Geometry: final body of the model. Coordinates: model frame, mm. A direction names the side the tool comes from. Round coordinates to 2 decimals unless told otherwise and drop trailing zeros. Write each loop counter-clockwise with the first axis right and the second up, starting at its lowest first coordinate (ties: lowest second). Pieces come first, ordered by that corner, then holes. Notation, with made-up numbers: (66, 53.25) - (110, 53.25) arc R8 cw to (110, 62.25) - close; hole circle Ø2 at (89, 0.5). An arc over 180 degrees is marked (long way). Write each question's results on one line, items separated by ' | '.
from build123d import *

# Parameters (mm, degrees)
EXTRUDE_1_DEPTH = 0.8
FILLET_1_R      = 4
FILLET_2_R      = 2


with BuildPart() as part:
    # 草图1 → 凸台-拉伸1 (new body)
    with BuildSketch(Plane(origin=(0, 0, 0), x_dir=(1, 0, 0), z_dir=(0, 1, 0))):
        with BuildLine():
            ThreePointArc((1.559359784, 16.778866316), (1.803429124, 18.895886668), (0, 20.03122292))
            Line((0, 20.03122292), (0, 18.83122292))
            ThreePointArc((0, 18.83122292), (0.8, 18.03122292), (0, 17.23122292))
            Line((0, 17.23122292), (0, 15.142135624))
            ThreePointArc((0, 15.142135624), (1, 14.142135624), (0, 13.142135624))
            Line((0, 13.142135624), (0, 12.142135624))
            Line((0, 12.142135624), (7.708712153, 11))
            ThreePointArc((7.708712153, 11), (7.543556444, 9.535365676), (8.232233047, 8.232233047))
            Line((8.232233047, 8.232233047), (9.292893219, 9.292893219))
            ThreePointArc((9.292893219, 9.292893219), (9.292893219, 10.707106781), (10.707106781, 10.707106781))
            Line((10.707106781, 10.707106781), (11.767766953, 11.767766953))
            ThreePointArc((11.767766953, 11.767766953), (9.864121635, 12.496304683), (8.05080027, 11.565445755))
            Line((8.05080027, 11.565445755), (1.559359784, 16.778866316))
        make_face()
    extrude_1 = extrude(amount=EXTRUDE_1_DEPTH)

    # 镜向1: 凸台-拉伸1 across plane
    add(extrude_1.mirror(Plane(origin=(0, 0.8, 0), x_dir=(-0.707106781, 0, 0.707106781), z_dir=(-0.707106781, 0, -0.707106781))))

    # 镜向2: part across plane


with BuildPart() as part_1:
    add(part.part)
    add(part.part.mirror(Plane(origin=(0, 0.8, 0), x_dir=(0, 0, 1), z_dir=(1, 0, 0))))

    # 镜向3: part across plane


with BuildPart() as part_2:
    add(part_1.part)
    add(part_1.part.mirror(Plane(origin=(0, 0.8, 0), x_dir=(1, 0, 0), z_dir=(0, 0, 1))))

    # 圆角1
    fillet_1_edges = [part_2.edges().sort_by_distance(p)[0] for p in [
        (7.708712153, 0.4, 11),
        (11, 0.4, 7.708712153),
        (12.142135624, 0.4, 0),
        (0, 0.4, 12.142135624),
        (-7.708712153, 0.4, 11),
        (-11, 0.4, 7.708712153),
        (-12.142135624, 0.4, 0),
        (7.708712153, 0.4, -11),
        (11, 0.4, -7.708712153),
        (0, 0.4, -12.142135624),
        (-7.708712153, 0.4, -11),
        (-11, 0.4, -7.708712153),
    ]]
    fillet(fillet_1_edges, radius=FILLET_1_R)

    # 圆角2
    fillet_2_edges = [part_2.edges().sort_by_distance(p)[0] for p in [
        (8.05080027, 0.4, 11.565445755),
        (1.559359784, 0.4, 16.778866316),
        (-1.559359784, 0.4, 16.778866316),
        (16.778866316, 0.4, 1.559359784),
        (11.565445755, 0.4, 8.05080027),
        (-11.565445755, 0.4, 8.05080027),
        (-8.05080027, 0.4, 11.565445755),
        (-16.778866316, 0.4, 1.559359784),
        (1.559359784, 0.4, -16.778866316),
        (8.05080027, 0.4, -11.565445755),
        (16.778866316, 0.4, -1.559359784),
        (11.565445755, 0.4, -8.05080027),
        (-8.05080027, 0.4, -11.565445755),
        (-1.559359784, 0.4, -16.778866316),
        (-16.778866316, 0.4, -1.559359784),
        (-11.565445755, 0.4, -8.05080027),
    ]]
    fillet(fillet_2_edges, radius=FILLET_2_R)


solid = part_2.part
Q1. Section query A-A, the plane z = 10. Return loops of the section in (x, y).
Answer block:
outline: (-12.5, 0) - (-11, 0) - (-11, 0.8) - (-12.5, 0.8) - close; (-9, 0) - (-7.12, 0) - (-7.12, 0.8) - (-9, 0.8) - close; (7.12, 0) - (9, 0) - (9, 0.8) - (7.12, 0.8) - close; (11, 0) - (12.5, 0) - (12.5, 0.8) - (11, 0.8) - close
Q2. Section query B-B, the plane x = 10. Return loops of the section in (y, z), plus the area to 3 significant figures.
Answer block:
outline: (0, -12.5) - (0.8, -12.5) - (0.8, -11) - (0, -11) - close; (0, -9) - (0.8, -9) - (0.8, -7.12) - (0, -7.12) - close; (0, 7.12) - (0.8, 7.12) - (0.8, 9) - (0, 9) - close; (0, 11) - (0.8, 11) - (0.8, 12.5) - (0, 12.5) - close | area: 5.40 mm2
Q3. Section query C-C, the plane z = -3.5. Return loops of the section in (x, y).
Answer block:
outline: (-15.22, 0) - (-11.62, 0) - (-11.62, 0.8) - (-15.22, 0.8) - close; (11.62, 0) - (15.22, 0) - (15.22, 0.8) - (11.62, 0.8) - close
Q4. Access query for faces 4 (the cylindrical face through (6.479, 0.406, 10.643)), 5 (the flat face through (14.17, 0.39, 4.81)). Directions: +Z, -Z, +X, -X, +Y, -Y. A direction counts if a zero-diameter tool reaches every point of the face in a straight line with its end or side. Return the directions, or none.
Answer block:
face 4: +Y, -Y | face 5: +Z, +X, +Y, -Y
Q5. Mould query, pull axis Z, two halves, no side actions, for faces 1 (the cylindrical face through (-10.643, 0.406, 6.479)), 2 (the flat face through (-2, 0, -12)), 3 (the flat face through (-14.17, 0.39, 4.81)). Classes: pulls with the +Z half, pulls with the -Z half, needs draft (parallel to the pull), parting line crosses it, or undercut.
Answer block:
face 1: undercut | face 2: needs draft | face 3: pulls with the +Z half
Q6. Ray query, line 1 along X through (y, z) = (0.5, 0); line 2 along Z through (x, y) = (10, 0.3); line 3 along X through (y, z) = (0.35, 18). Return the intervals inside material, ascending.
Answer block:
line 1: -20.03 to -18.83, -17.23 to -15.14, -13.14 to -12.1, 12.1 to 13.14, 15.14 to 17.23, 18.83 to 20.03 | line 2: -12.5 to -11, -9 to -7.12, 7.12 to 9, 11 to 12.5 | line 3: -2 to -0.8, 0.8 to 2
Q7. Section query D-D, the plane y = 0.45. Give the number of separate pieces and of enclosed holes in the cut face, plus the area to 3 significant figures.
Answer block:
separate pieces: 1 | enclosed holes: 13 | area: 307 mm2
